Verification items for this drawing (mm, ordinates from the low corner). A direction names the side the tool comes from. Give positions to 0.01 mm unless a question says otherwise; leave off trailing zeros. Loops run counter-clockwise (first coordinate to the right, second up) from the corner with the lowest first, then second, coordinate; pieces in that order, holes last. Notation, with made-up numbers: (14, -15.75) -> (43, -15.75) arc R22 ccw to (43, -0.75) -> close; hole circle Ø5 at (55, 62). An arc over 180 degrees is marked (long way). Answer in a Markdown table with one row per item. Add a question column.
Q1. Section check D-D on y = 3. Enter the section's corners in (x, z) (1 decimal), and give its area (3 significant figures).
Q2. Section check A-A on y = 6.75. Enter the section's corners in (x, z) (1 decimal), and give its area (3 significant figures).
Q3. Section check B-B on x = 4. Enter the section's corners in (y, z).
Q4. Release check for a two-part mould opening along X. For the marked faces 1, 2, 3 and 4 record: pulls with the +X half, pulls with the -X half, needs draft (parallel to the pull), parting line crosses it, or undercut.
Q5. Material ranges on probe 1 along Z at (x, y) = (52, 7); probe 2 along X at (y, z) = (7.5, 3.75) (1 decimal); probe 3 along X at (y, z) = (13.25, 15), recorded low to high.
Q6. Section check C-C on z = 15. Enter the section's corners in (x, y).
Q7. Set-up check for the marked faces 5 and 6: record each of +Z, -Z, +X, -X, +Y, -Y from which the full face is reachable in a straight line by a thin tool's end or side.
Q8. Gauge pin test, flat ends, axial feed: P1, Ø8, axis at y = 23, z = 2, coming from the -X side; P2, Ø2, axis at x = 45, z = 16.5, coming from the +Y side; P3, Ø2.5, axis at x = 3.5, z = 4.5, coming from the +Y side; P4, Ø5, axis at x = 52, z = 15, coming from the -Y side. Record the tip position at first contact, or that the pin passes through.
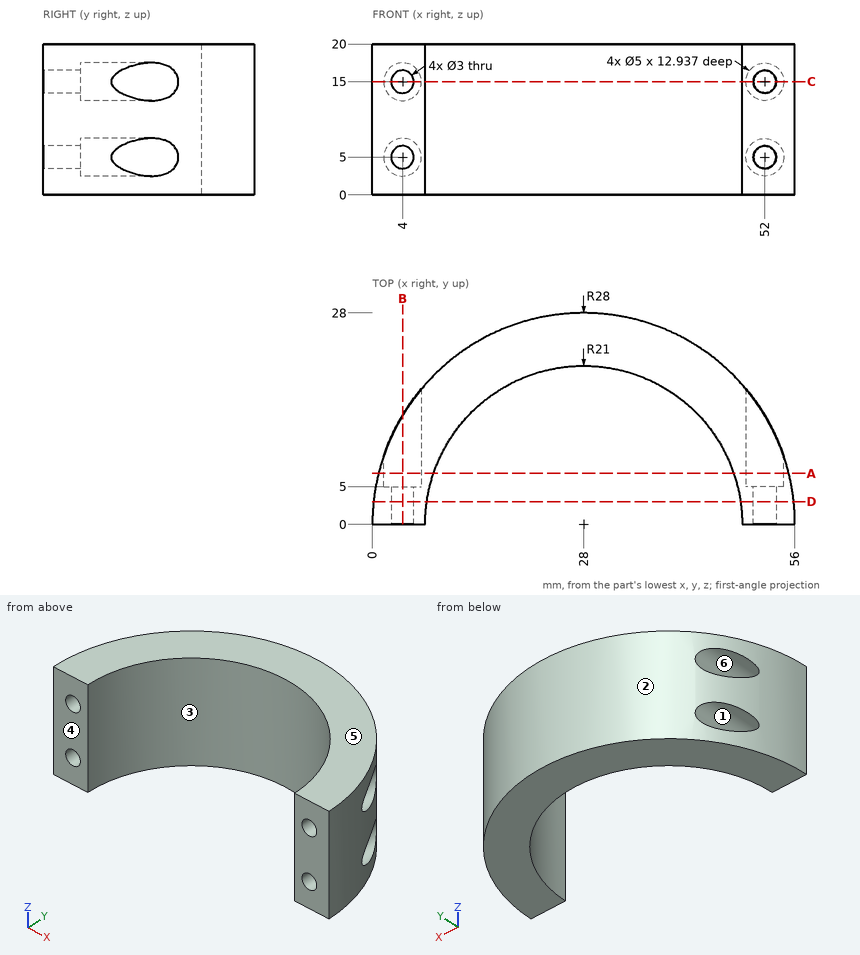
Taken from the geometry:
| question | item | result |
|---|---|---|
| 1 | outline | (0.2, 0) -> (7.2, 0) -> (7.2, 20) -> (0.2, 20) -> close; (48.8, 0) -> (55.8, 0) -> (55.8, 20) -> (48.8, 20) -> close; hole circle Ø3 at (4, 5); hole circle Ø3 at (4, 15); hole circle Ø3 at (52, 5); hole circle Ø3 at (52, 15) |
| 1 | area | 254 mm² |
| 2 | outline | (0.8, 0) -> (8.1, 0) -> (8.1, 20) -> (0.8, 20) -> close; (47.9, 0) -> (55.2, 0) -> (55.2, 20) -> (47.9, 20) -> close; hole circle Ø5 at (4, 5); hole circle Ø5 at (4, 15); hole circle Ø5 at (52, 5); hole circle Ø5 at (52, 15) |
| 2 | area | 213 mm² |
| 3 | outline | (0, 0) -> (14.42, 0) -> (14.42, 2.5) -> (5, 2.5) -> (5, 3.5) -> (0, 3.5) -> close; (0, 6.5) -> (5, 6.5) -> (5, 7.5) -> (14.42, 7.5) -> (14.42, 12.5) -> (5, 12.5) -> (5, 13.5) -> (0, 13.5) -> close; (0, 16.5) -> (5, 16.5) -> (5, 17.5) -> (14.42, 17.5) -> (14.42, 20) -> (0, 20) -> close |
| 4 | face 1 | undercut |
| 4 | face 2 | parting line crosses it |
| 4 | face 3 | undercut |
| 4 | face 4 | needs draft |
| 5 | probe 1 | z = 0 to 2.5, 7.5 to 12.5, 17.5 to 20 |
| 5 | probe 2 | x = 1 to 1.8, 6.2 to 8.4, 47.6 to 49.8, 54.2 to 55 |
| 5 | probe 3 | x = 6.5 to 11.71, 44.29 to 49.5 |
| 6 | outline | (0, 0) -> (2.5, 0) -> (2.5, 5) -> (1.5, 5) -> (1.5, 9.04) arc R28 ccw to start; (5.5, 0) -> (7, 0) arc R21 cw to (49, 0) -> (50.5, 0) -> (50.5, 5) -> (49.5, 5) -> (49.5, 17.94) arc R28 ccw to (6.5, 17.94) -> (6.5, 5) -> (5.5, 5) -> close; (53.5, 0) -> (56, 0) arc R28 ccw to (54.5, 9.04) -> (54.5, 5) -> (53.5, 5) -> close |
| 7 | face 5 | +Z, +X, -X, +Y, -Y |
| 7 | face 6 | +Y |
| 8 | P1 | stops at x = 7.43 |
| 8 | P2 | stops at y = 22.98 |
| 8 | P3 | stops at y = 5 |
| 8 | P4 | stops at y = 0 |
